from build123d import *

# Parameters (mm, degrees)
F0_R     = 11.3
F1_DEPTH = 7
F2_R     = 2


# Not quite as in the source:
# - a feature names something its author has since deleted; it is built from what else it names


with BuildPart() as f1:
    # F0 (on Top) → F1 (new body)
    with BuildSketch(Plane.XY):
        with BuildLine():
            Line((8.8875694593, 38.6650469228), (6.5895106012, 33.0585853257))
            ThreePointArc((6.5895106012, 33.0585853257), (26.0616292761, 21.3795040442), (33.7089263208, 0))
            ThreePointArc((33.7089263208, 0), (23.6957200597, -23.9750821594), (-0.3950708864, -33.7066111126))
            Line((-0.3950708864, -33.7066111126), (-4.7252705017, -39.390945192))
            ThreePointArc((-4.7252705017, -39.390945192), (26.3297116519, -29.6769443973), (39.6733505572, 0))
            ThreePointArc((39.6733505572, 0), (31.0368684244, 24.7120930485), (8.8875694593, 38.6650469228))
        make_face()
        with BuildLine():
            ThreePointArc((0.6589035842, 33.7024859583), (3.6384789483, 33.5119856864), (6.5895106012, 33.0585853257))
            Line((6.5895106012, 33.0585853257), (8.8875694593, 38.6650469228))
            ThreePointArc((8.8875694593, 38.6650469228), (6.2429099817, 39.1790865053), (3.5694610238, 39.5124498409))
            Line((3.5694610238, 39.5124498409), (0.6589035842, 33.7024859583))
        make_face()
        with BuildLine():
            Line((-10.061211071, -38.3763830528), (-6.8087075048, -33.0141366056))
            ThreePointArc((-6.8087075048, -33.0141366056), (-33.4997306504, 3.7496346558), (0.6589035842, 33.7024859583))
            Line((0.6589035842, 33.7024859583), (3.5694610238, 39.5124498409))
            ThreePointArc((3.5694610238, 39.5124498409), (-39.0794482696, 6.8389668354), (-10.061211071, -38.3763830528))
        make_face()
        with BuildLine():
            ThreePointArc((-0.3950708864, -33.7066111126), (-3.6184922292, -33.5141496638), (-6.8087075048, -33.0141366056))
            Line((-6.8087075048, -33.0141366056), (-10.061211071, -38.3763830528))
            ThreePointArc((-10.061211071, -38.3763830528), (-7.4106236855, -38.9750869277), (-4.7252705017, -39.390945192))
            Line((-4.7252705017, -39.390945192), (-0.3950708864, -33.7066111126))
        make_face()
        with BuildLine():
            ThreePointArc((3.5694610238, 39.5124498409), (6.2429099817, 39.1790865053), (8.8875694593, 38.6650469228))
            Line((8.8875694593, 38.6650469228), (6.4280834783, 45.2187427282))
            Line((6.4280834783, 45.2187427282), (3.5694610238, 39.5124498409))
        make_face()
        with BuildLine():
            ThreePointArc((-4.7252705017, -39.390945192), (-7.4106236855, -38.9750869277), (-10.061211071, -38.3763830528))
            Line((-10.061211071, -38.3763830528), (-8.8514386924, -44.8074434017))
            Line((-8.8514386924, -44.8074434017), (-4.7252705017, -39.390945192))
        make_face()
        with BuildLine():
            ThreePointArc((-9.0146919562, 14.392356585), (-4.6897069772, 16.3221091653), (0, 16.9824791811))
            Line((0, 16.9824791811), (6.5895106012, 33.0585853257))
            ThreePointArc((6.5895106012, 33.0585853257), (3.6384789483, 33.5119856864), (0.6589035842, 33.7024859583))
            Line((0.6589035842, 33.7024859583), (-9.0146919562, 14.392356585))
        make_face()
        with BuildLine():
            ThreePointArc((3.0870048037, -16.6995509065), (13.054301857, -10.8623110875), (16.9824791811, 0))
            ThreePointArc((16.9824791811, 0), (12.0084261903, 12.0084261903), (0, 16.9824791811))
            ThreePointArc((0, 16.9824791811), (-4.6897069772, 16.3221091653), (-9.0146919562, 14.392356585))
            ThreePointArc((-9.0146919562, 14.392356585), (-15.7401759471, 6.37584977), (-16.4896996402, -4.0613304363))
            ThreePointArc((-16.4896996402, -4.0613304363), (-14.690740637, -8.5197851306), (-11.7143980752, -12.2954250382))
            ThreePointArc((-11.7143980752, -12.2954250382), (-4.8432488922, -16.2772091989), (3.0870048037, -16.6995509065))
        make_face()
        Circle(F0_R, mode=Mode.SUBTRACT)
        with BuildLine():
            Line((-20.9624820809, -13.7546608704), (-11.7143980752, -12.2954250382))
            ThreePointArc((-11.7143980752, -12.2954250382), (-14.690740637, -8.5197851306), (-16.4896996402, -4.0613304363))
            Line((-16.4896996402, -4.0613304363), (-20.9624820809, -13.7546608704))
        make_face()
        with BuildLine():
            Line((28.1798244973, 3.8041888679), (16.9824791811, 0))
            ThreePointArc((16.9824791811, 0), (13.054301857, -10.8623110875), (3.0870048037, -16.6995509065))
            Line((3.0870048037, -16.6995509065), (-6.8087075048, -33.0141366056))
            ThreePointArc((-6.8087075048, -33.0141366056), (-3.6184922292, -33.5141496638), (-0.3950708864, -33.7066111126))
            Line((-0.3950708864, -33.7066111126), (28.1798244973, 3.8041888679))
        make_face()
    extrude(amount=F1_DEPTH)

    # F2
    f2_edges = [f1.edges().sort_by_distance(p)[0] for p in [
        (39.083445, -6.81609, 7),
        (39.083445, -6.81609, 0),
        (-39.079448, 6.838967, 0),
        (-39.079448, 6.838967, 7),
    ]]
    fillet(f2_edges, radius=F2_R)


solid = f1.part
Can you work these out from the model? Positions are in its coordinate system, mm. A direction names the side the tool comes from. Give positions to 0.01 mm unless a question says otherwise; leave off trailing zeros. Return JSON: item names as keys, results as strings.
1. I want a section at B-B on y = 28. Give the number of separate pieces and of enclosed holes in the cut face, and give its area (3 significant figures).
Output values:
{"separate pieces": "3", "enclosed holes": "0", "area": "173 mm²"}
2. We'd pull the mould along X, two halves only. Please class faces 1 (the face through (-9.493, -41.395, 3.451)), 2 (the face through (5.4, 10.4, 0)), 3 (the face through (-33.57, 3.06, 3.45)): +X half, -X half, draft (parallel to the pull), parting line (faces both ways), or undercut.
Output values:
{"face 1": "-X half", "face 2": "draft", "face 3": "undercut"}
3. If I drill on line 1 (X direction, y = -1, z = 3.25); line 2 (Y direction, x = -19.5, z = 6.75); line 3 (X direction, y = -15.5, z = 3.75), over which ranges is the centre line in solid material (lowest first)?
Output values:
{"line 1": "x = -39.66 to -33.69, -16.95 to -11.26, 11.26 to 24.52, 33.69 to 39.66", "line 2": "y = -33.36 to -27.5, -13.52 to -10.59, 27.5 to 33.36", "line 3": "x = -36.52 to -29.93, -6.94 to 13.47, 29.93 to 36.52"}
4. For faces 4 (the face through (5.4, 10.4, 7)), 5 (the face through (-16.403, -13.035, 3.451)), which set-ups out of +Z, -Z, +X, -X, +Y, -Y let a thin tool reach every point of the face, with its end or its side?
Output values:
{"face 4": "+Z, +X, -X, +Y, -Y", "face 5": "+Z, -Z"}
5. I'm going to push flat-ended pins straight in: pin 1 Ø3 at (x, z) = (-18.5, 4.5) entering from -Y; pin 2 Ø3 at (y, z) = (22.5, 1.5) entering from -X; pin 3 Ø4 at (x, z) = (2, 6) entering from +Y. Where does each tip first touch, or does it pass through?
Output values:
{"pin 1": "stops at y = -35.85", "pin 2": "stops at x = -33.63", "pin 3": "stops at y = 40.37"}
